Verification items for the finished model (mm, model axes). Face numbers are marked on the shaded views. A direction names the side the tool comes from. Give positions to 0.01 mm unless a question says otherwise; leave off trailing zeros.
from build123d import *

# Parameters (mm, degrees)
F0_R     = 38.1
F0_R_2   = 36.386913731
F1_DEPTH = 12.7
F2_R     = 1.5
F4_DEPTH = 12.7
F0_R_3   = 34.925
F5_DEPTH = 9.525
F7_DEPTH = 9.525
F9_DEPTH = 9.525


with BuildPart() as f1:
    # F0 (on Front) → F1 (new body, symmetric)
    with BuildSketch(Plane.XZ):
        Circle(F0_R)
        Circle(F0_R_2, mode=Mode.SUBTRACT)
    extrude(amount=F1_DEPTH, both=True)

    # F2
    f2_edges = [f1.edges().sort_by_distance(p)[0] for p in [
        (-38.1, -12.7, 0),
        (-38.1, 12.7, 0),
    ]]
    fillet(f2_edges, radius=F2_R)

    # F3 (on Front) → F4 (join, symmetric)
    with BuildSketch(Plane.XZ):
        Polygon((-11.8081336841, -8.5378140211), (-26.464993082, -25.2349018068), (4.8301340017, -1.8485224727), (-3.5016993061, -3.3492420334), (15.7506130636, 12.5613436103), (6.9332248531, 11.4183481783), (24.5728250593, 25.4238694906), (4.1189347394, 19.9994817376), (-10.358533822, 3.8266193587), (-2.5237547234, 5.047195591), (-17.8205184639, -9.6808085218), align=None)
    extrude(amount=F4_DEPTH, both=True)

    # F0 (on Front) → F5 (join, symmetric)
    with BuildSketch(Plane.XZ):
        Circle(F0_R_2)
        Circle(F0_R_3, mode=Mode.SUBTRACT)
    extrude(amount=F5_DEPTH, both=True)

    # F6 (on Front) → F7 (join, symmetric)
    with BuildSketch(Plane.XZ):
        with BuildLine():
            Line((-19.0900918096, -17.018487677), (-16.3832232356, -13.7969218194))
            add(Edge.make_bspline(
                [(-16.3832232356, -13.7969218194), (-25.3736051563, -9.473731392), (-29.0905786368, 8.1572549104), (-7.3840054694, 19.1332485124), (2.8318234254, 18.4940695763)],
                knots=[0, 0, 0, 0, 0.4527371046, 1, 1, 1, 1], degree=3))
            Line((2.8318234254, 18.4940695763), (4.588526208, 20.0228095055))
            add(Edge.make_bspline(
                [(-19.0900918096, -17.018487677), (-28.620544821, -11.2098539248), (-29.5136057934, 10.2947418894), (-6.1136707664, 20.5405261368), (4.588526208, 20.0228095055)],
                knots=[0, 0, 0, 0, 0.4639479817, 1, 1, 1, 1], degree=3))
        make_face()
    extrude(amount=F7_DEPTH, both=True)

    # F8 (on Front) → F9 (join, symmetric)
    with BuildSketch(Plane.XZ):
        with BuildLine():
            add(Edge.make_bspline(
                [(-13.784956187, -14.9299576879), (-0.5538631669, -18.623918621), (24.9938380842, -8.3206427927), (23.5522668809, 11.1457686871), (13.0951637402, 16.5083874017)],
                knots=[0, 0, 0, 0, 0.5594726936, 1, 1, 1, 1], degree=3))
            Line((-13.784956187, -14.9299576879), (-17.4717549235, -18.0134642869))
            add(Edge.make_bspline(
                [(-17.4717549235, -18.0134642869), (-0.7163750913, -25.6539166477), (35.1580871339, -8.4938520858), (26.0995104909, 13.357847929), (14.8380147293, 18.3182712644)],
                knots=[0, 0, 0, 0, 0.5723759264, 1, 1, 1, 1], degree=3))
            Line((14.8380147293, 18.3182712644), (13.0951637402, 16.5083874017))
        make_face()
    extrude(amount=F9_DEPTH, both=True)


solid = f1.part
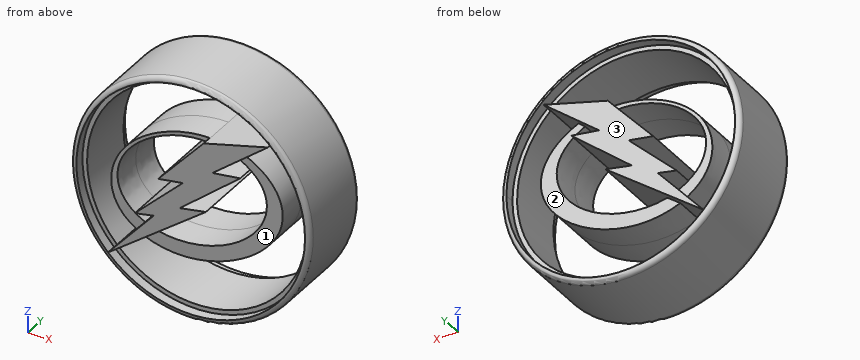
(1) Go/stop test with flat-tipped pins: pin 1 (4 mm diameter, centred on y = 0.5, z = 7.5, fed in from +X); pin 2 (10 mm diameter, centred on x = -11, z = -25, fed in from +Y) (3 decimals); pin 3 (1.5 mm diameter, centred on y = 8.5, z = 15.5, fed in from -X). Record where each tip stops, or that it passes through.
Solved:
pin 1: stops at x = 37.7
pin 2: stops at y = 9.525
pin 3: stops at x = -35.13
(2) Scan lines: line 1 (Z direction, x = 0, y = -10.6); line 2 (Z direction, x = -4.5, y = -3); line 3 (X direction, y = 7.25, z = -23). Record each from-to range of solid material in increasing order.
Solved:
line 1: z = -38.1 to -36.39, -5.46 to -2.72, -0.46 to 15.4, 36.39 to 38.1
line 2: z = -37.83 to -34.63, -20.72 to -16.06, -8.82 to 3.14, 4.74 to 10.37, 17.91 to 19.14, 34.63 to 37.83
line 3: x = -30.37 to -26.28, -24.5 to -23.47, 26.28 to 30.37
(3) Section check A-A, the plane x = 18. Give the number of separate pieces and of enclosed holes in the cut face, then the cut area to 3 significant figures.
Solved:
separate pieces: 5
enclosed holes: 0
area: 447 mm2
(4) Set-up check for the marked faces 1, 2 and 3: record each of +Z, -Z, +X, -X, +Y, -Y from which the full face is reachable in a straight line by a thin tool's end or side.
Solved:
face 1: -Y
face 2: +Y
face 3: +Z, -Z, +X, -X, +Y
